Geometry check sheet. Reference: the model listing, model coordinates, mm. Give positions to 0.01 mm unless a question says otherwise; leave off trailing zeros. Order: outer loops, then holes, each group sorted by start corner. A loop starts at its lowest first (then second) coordinate and runs counter-clockwise, first axis right, second up. Notation, with made-up numbers: M 23.5,13 L 59.5,13 A30 cw 59.5,39 Z; hole C -33.5,9.25 d10. An arc over 180 degrees is marked long. Use CSV: the item, a comma, the result in double quotes. Start each with the question number.
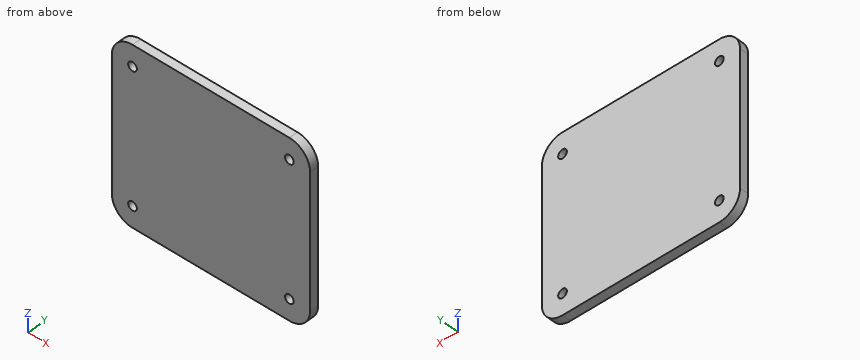
from build123d import *

# Parameters (mm, degrees)
BOSS_EXTRUDE1_DEPTH = 3.175


with BuildPart() as part:
    # Sketch1 → Boss-Extrude1 (new body)
    with BuildSketch(Plane(origin=(0, 0, 0), x_dir=(1, 0, 0), z_dir=(0, 1, 0))):
        with BuildLine():
            Line((-92.0838, 72.2973), (-34.9338, 72.2973))
            ThreePointArc((-34.9338, 72.2973), (-29.60221487, 74.50571487), (-27.3938, 79.8373))
            Line((-27.3938, 79.8373), (-27.3938, 128.0973))
            ThreePointArc((-27.3938, 128.0973), (-29.60221487, 133.42888513), (-34.9338, 135.6373))
            Line((-34.9338, 135.6373), (-92.0838, 135.6373))
            ThreePointArc((-92.0838, 135.6373), (-97.41538513, 133.42888513), (-99.6238, 128.0973))
            Line((-99.6238, 128.0973), (-99.6238, 79.8373))
            ThreePointArc((-99.6238, 79.8373), (-97.41538513, 74.50571487), (-92.0838, 72.2973))
        make_face()
        with BuildLine():
            add(Edge.make_bspline(
                [(-33.3463, 79.8373), (-33.3463, 80.7141), (-34.057, 81.4248), (-34.9338, 81.4248)],
                knots=[0, 0, 0, 0, 0.2, 0.2, 0.2, 0.2], degree=3))
            add(Edge.make_bspline(
                [(-34.9338, 81.4248), (-35.8106, 81.4248), (-36.5213, 80.7141), (-36.5213, 79.8373)],
                knots=[0.2, 0.2, 0.2, 0.2, 0.4, 0.4, 0.4, 0.4], degree=3))
            add(Edge.make_bspline(
                [(-36.5213, 79.8373), (-36.5213, 78.9605), (-35.8106, 78.2498), (-34.9338, 78.2498)],
                knots=[0.4, 0.4, 0.4, 0.4, 0.6, 0.6, 0.6, 0.6], degree=3))
            add(Edge.make_bspline(
                [(-34.9338, 78.2498), (-34.057, 78.2498), (-33.3463, 78.9605), (-33.3463, 79.8373)],
                knots=[0.6, 0.6, 0.6, 0.6, 1, 1, 1, 1], degree=3))
        make_face(mode=Mode.SUBTRACT)
        with BuildLine():
            add(Edge.make_bspline(
                [(-33.3463, 128.0973), (-33.3463, 128.9741), (-34.057, 129.6848), (-34.9338, 129.6848)],
                knots=[0, 0, 0, 0, 0.2, 0.2, 0.2, 0.2], degree=3))
            add(Edge.make_bspline(
                [(-34.9338, 129.6848), (-35.8106, 129.6848), (-36.5213, 128.9741), (-36.5213, 128.0973)],
                knots=[0.2, 0.2, 0.2, 0.2, 0.4, 0.4, 0.4, 0.4], degree=3))
            add(Edge.make_bspline(
                [(-36.5213, 128.0973), (-36.5213, 127.2205), (-35.8106, 126.5098), (-34.9338, 126.5098)],
                knots=[0.4, 0.4, 0.4, 0.4, 0.6, 0.6, 0.6, 0.6], degree=3))
            add(Edge.make_bspline(
                [(-34.9338, 126.5098), (-34.057, 126.5098), (-33.3463, 127.2205), (-33.3463, 128.0973)],
                knots=[0.6, 0.6, 0.6, 0.6, 1, 1, 1, 1], degree=3))
        make_face(mode=Mode.SUBTRACT)
        with BuildLine():
            add(Edge.make_bspline(
                [(-90.4963, 128.0973), (-90.4963, 128.9741), (-91.207, 129.6848), (-92.0838, 129.6848)],
                knots=[0, 0, 0, 0, 0.2, 0.2, 0.2, 0.2], degree=3))
            add(Edge.make_bspline(
                [(-92.0838, 129.6848), (-92.9606, 129.6848), (-93.6713, 128.9741), (-93.6713, 128.0973)],
                knots=[0.2, 0.2, 0.2, 0.2, 0.4, 0.4, 0.4, 0.4], degree=3))
            add(Edge.make_bspline(
                [(-93.6713, 128.0973), (-93.6713, 127.2205), (-92.9606, 126.5098), (-92.0838, 126.5098)],
                knots=[0.4, 0.4, 0.4, 0.4, 0.6, 0.6, 0.6, 0.6], degree=3))
            add(Edge.make_bspline(
                [(-92.0838, 126.5098), (-91.207, 126.5098), (-90.4963, 127.2205), (-90.4963, 128.0973)],
                knots=[0.6, 0.6, 0.6, 0.6, 1, 1, 1, 1], degree=3))
        make_face(mode=Mode.SUBTRACT)
        with BuildLine():
            add(Edge.make_bspline(
                [(-90.4963, 79.8373), (-90.4963, 80.7141), (-91.207, 81.4248), (-92.0838, 81.4248)],
                knots=[0, 0, 0, 0, 0.2, 0.2, 0.2, 0.2], degree=3))
            add(Edge.make_bspline(
                [(-92.0838, 81.4248), (-92.9606, 81.4248), (-93.6713, 80.7141), (-93.6713, 79.8373)],
                knots=[0.2, 0.2, 0.2, 0.2, 0.4, 0.4, 0.4, 0.4], degree=3))
            add(Edge.make_bspline(
                [(-93.6713, 79.8373), (-93.6713, 78.9605), (-92.9606, 78.2498), (-92.0838, 78.2498)],
                knots=[0.4, 0.4, 0.4, 0.4, 0.6, 0.6, 0.6, 0.6], degree=3))
            add(Edge.make_bspline(
                [(-92.0838, 78.2498), (-91.207, 78.2498), (-90.4963, 78.9605), (-90.4963, 79.8373)],
                knots=[0.6, 0.6, 0.6, 0.6, 1, 1, 1, 1], degree=3))
        make_face(mode=Mode.SUBTRACT)
    extrude(amount=BOSS_EXTRUDE1_DEPTH)


solid = part.part
(1) Sectioned sample at A-A on y = 2.65. Give the number of separate pieces and of enclosed holes in the cut face, then the cut area to 3 significant figures.
(2) Sectioned sample at B-B on x = -32. Record the cut outline in (y, z) (3 decimals), then the cut area to 3 significant figures.
(3) Thickness scan on line 1 (X direction, y = 0.5, z = -78); line 2 (X direction, y = 1, z = -77). Record the ranges inside material, lowest first.
Responses:
1,separate pieces,"1"
1,enclosed holes,"4"
1,area,"4,490 mm2"
2,outline,"M 0,-135.043 L 3.175,-135.043 L 3.175,-72.891 L 0,-72.891 Z"
2,area,"197 mm2"
3,line 1,"-99.4 to -27.62"
3,line 2,"-99.07 to -27.95"
